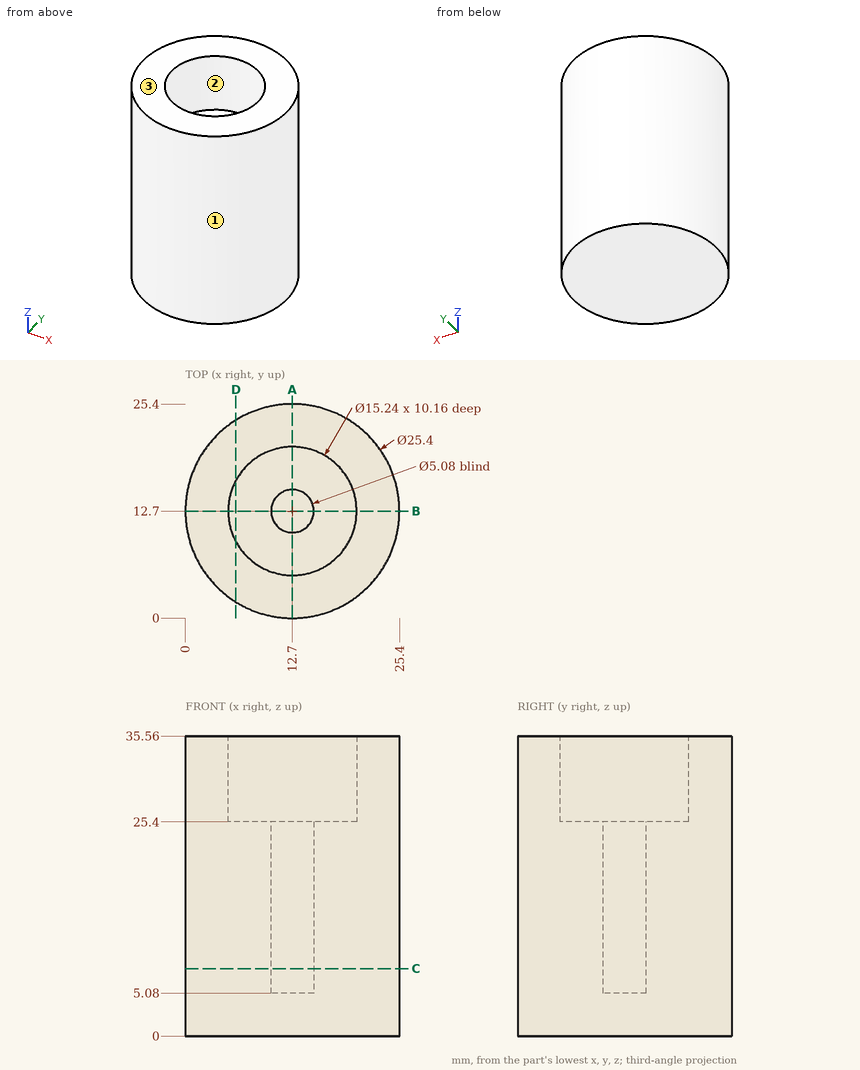
Geometry check sheet. Reference: drawing and pictorial views, mm from the part's lowest x, y, z. Give positions to 0.01 mm unless a question says otherwise; leave off trailing zeros. Write each loop counter-clockwise with the first axis right and the second up, starting at its lowest first coordinate (ties: lowest second). Pieces come first, ordered by that corner, then holes. Notation, with made-up numbers: M 51.25,-2.5 L 69.25,-2.5 A21 cw 69.25,10.5 Z; hole C -22.5,-13 d2. An arc over 180 degrees is marked long. Use CSV: the item, a comma, the result in double quotes.
1) Cross-section at D-D (x = 6). Enter the section's corners in (y, z), plus the area to 3 significant figures.
Final values:
outline,"M 1.91,0 L 23.49,0 L 23.49,35.56 L 16.33,35.56 L 16.33,25.4 L 9.07,25.4 L 9.07,35.56 L 1.91,35.56 Z"
area,"694 mm²"
2) Cross-section at A-A (x = 12.7). Enter the section's corners in (y, z), plus the area to 3 significant figures.
Final values:
outline,"M 0,0 L 25.4,0 L 25.4,35.56 L 20.32,35.56 L 20.32,25.4 L 15.24,25.4 L 15.24,5.08 L 10.16,5.08 L 10.16,25.4 L 5.08,25.4 L 5.08,35.56 L 0,35.56 Z"
area,"645 mm²"
3) Release check for a two-part mould opening along X. For the marked faces 1, 2 and 3 record: released by +X, released by -X, zero draft, split by the parting line, or undercut.
Final values:
face 1,"split by the parting line"
face 2,"undercut"
face 3,"zero draft"
4) Cross-section at C-C (z = 8). Enter the section's corners in (x, y), plus the area to 3 significant figures.
Final values:
outline,"C 12.7,12.7 d25.4; hole C 12.7,12.7 d5.08"
area,"486 mm²"
5) Go/stop test with flat-tipped pins: pin 1 Ø1.5 at (x, z) = (22, 16.5) entering from -Y; pin 2 Ø5.5 at (x, y) = (13, 13.5) entering from +Z; pin 3 Ø3 at (x, z) = (21, 26.5) entering from -Y. Record where each tip stops, or that it passes through.
Final values:
pin 1,"y = 3.31"
pin 2,"z = 25.4"
pin 3,"y = 1.97"
6) Material ranges on line 1 along Y through (x, z) = (12.7, 20); line 2 along Y through (x, z) = (12.7, 32); line 3 along Z through (x, y) = (6.25, 12), recorded low to high.
Final values:
line 1,"0 to 10.16, 15.24 to 25.4"
line 2,"0 to 5.08, 20.32 to 25.4"
line 3,"0 to 25.4"
